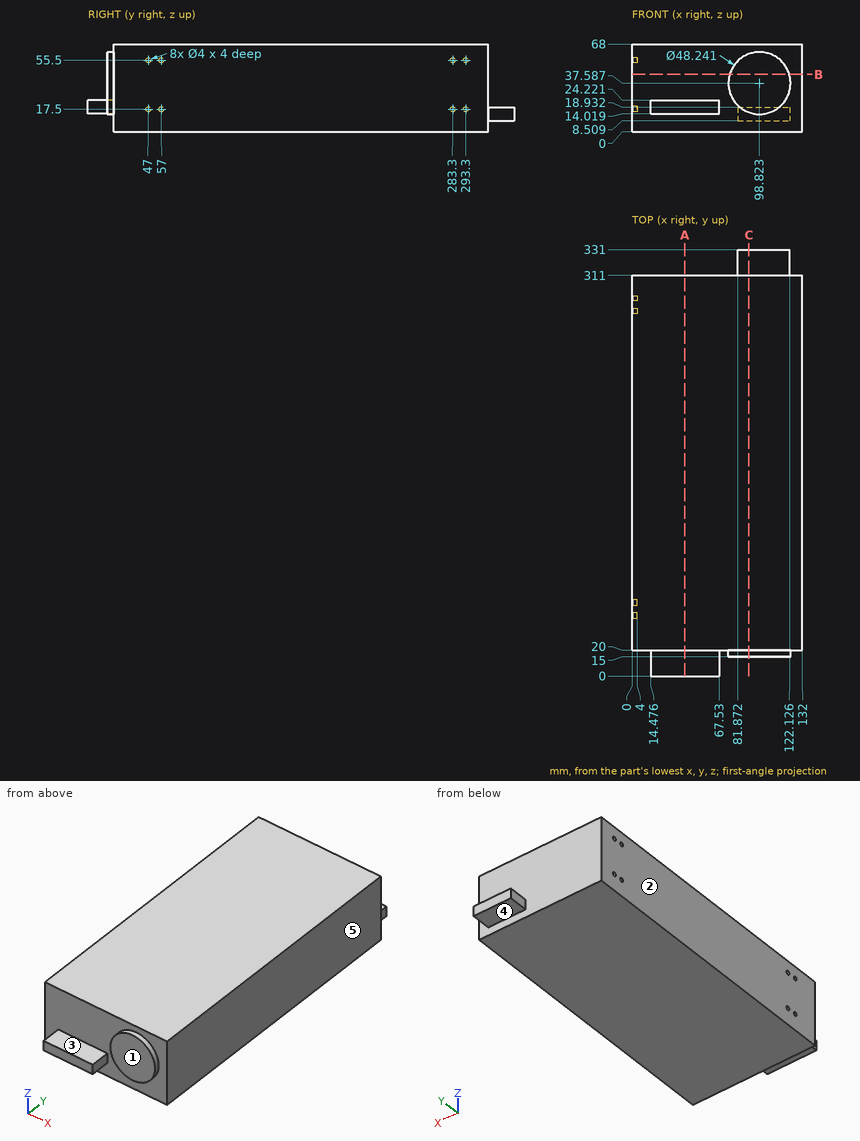
Check sheet for the drawn part. Datum: minimum x, y, z corner. Units: mm. A direction names the side the tool comes from. Round coordinates to 2 decimals unless told otherwise and drop trailing zeros. Loops run counter-clockwise (first coordinate to the right, second up) from the corner with the lowest first, then second, coordinate; pieces in that order, holes last. Notation, with made-up numbers: (-2.75, -20) -> (17.25, -20) arc R37 cw to (17.25, 17) -> close; hole circle Ø6 at (52.25, -8.5). An arc over 180 degrees is marked (long way). Put each result on its own line as item: value. Start each with the question number.
1. Section check A-A (x = 41). Enter the section's corners in (y, z), plus the area to 3 significant figures.
2. Access from +Z, -Z, +X, -X, +Y, -Y to the whole of each face (thin tool, end or side, straight path). Record for the marked faces 1, 2, 3, 4 and 5.
3. Gauge pin test, flat ends, axial feed: pin 1 (4 mm diameter, centred on x = 98.5, z = 37, fed in from +Y); pin 2 (10 mm diameter, centred on x = 60.5, z = 21, fed in from -Y); pin 3 (11 mm diameter, centred on y = 11.5, z = 18.5, fed in from -X); pin 4 (10 mm diameter, centred on x = 30.5, y = 5.5, fed in from -Z). Record the tip position at first contact, or that the pin passes through.
4. Section check C-C (x = 90.5). Enter the section's corners in (y, z), plus the area to 3 significant figures.
5. Section check B-B (z = 44.5). Enter the section's corners in (x, y), plus the area to 3 significant figures.
6. Scan lines: probe 1 along Z at (x, y) = (1.8, 57); probe 2 along Y at (x, z) = (1, 17); probe 3 along Z at (x, y) = (121.5, 315.5). Record each from-to range of solid material in increasing order.
Findings:
1. outline: (0, 14.02) -> (20, 14.02) -> (20, 0) -> (311, 0) -> (311, 68) -> (20, 68) -> (20, 24.22) -> (0, 24.22) -> close
1. area: 20,000 mm^2
2. face 1: +Z, -Z, +X, -Y
2. face 2: +Z, -Z, -X, +Y, -Y
2. face 3: +Z, -X, -Y
2. face 4: -Z, +X, -X, +Y
2. face 5: +Z, -Z, +X, +Y, -Y
3. pin 1: stops at y = 311
3. pin 2: stops at y = 0
3. pin 3: stops at x = 14.48
3. pin 4: stops at z = 14.02
4. outline: (15, 14.95) -> (20, 14.95) -> (20, 0) -> (311, 0) -> (311, 8.51) -> (331, 8.51) -> (331, 18.93) -> (311, 18.93) -> (311, 68) -> (20, 68) -> (20, 60.23) -> (15, 60.23) -> close
4. area: 20,200 mm^2
5. outline: (0, 20) -> (75.71, 20) -> (75.71, 15) -> (121.93, 15) -> (121.93, 20) -> (132, 20) -> (132, 311) -> (0, 311) -> close
5. area: 38,600 mm^2
6. probe 1: z = 0 to 15.5, 19.5 to 53.5, 57.5 to 68
6. probe 2: y = 20 to 45.06, 48.94 to 55.06, 58.94 to 281.36, 285.24 to 291.36, 295.24 to 311
6. probe 3: z = 8.51 to 18.93
